Input: dimensioned drawing with shaded views. Units: mm. Origin: part minimum x, y, z. A direction names the side the tool comes from. Give positions to 0.01 mm unless a question says otherwise; leave off trailing zeros. Write each loop counter-clockwise with the first axis right and the second up, starting at its lowest first coordinate (ties: lowest second). Pieces come first, ordered by that corner, then holes. Notation, with made-up numbers: M -22,78.5 L 14,78.5 A21 ccw 14,86.5 Z; hole C 18,-15.5 d9. An arc over 180 degrees is marked long. Answer as a JSON object with one key per item and string values.
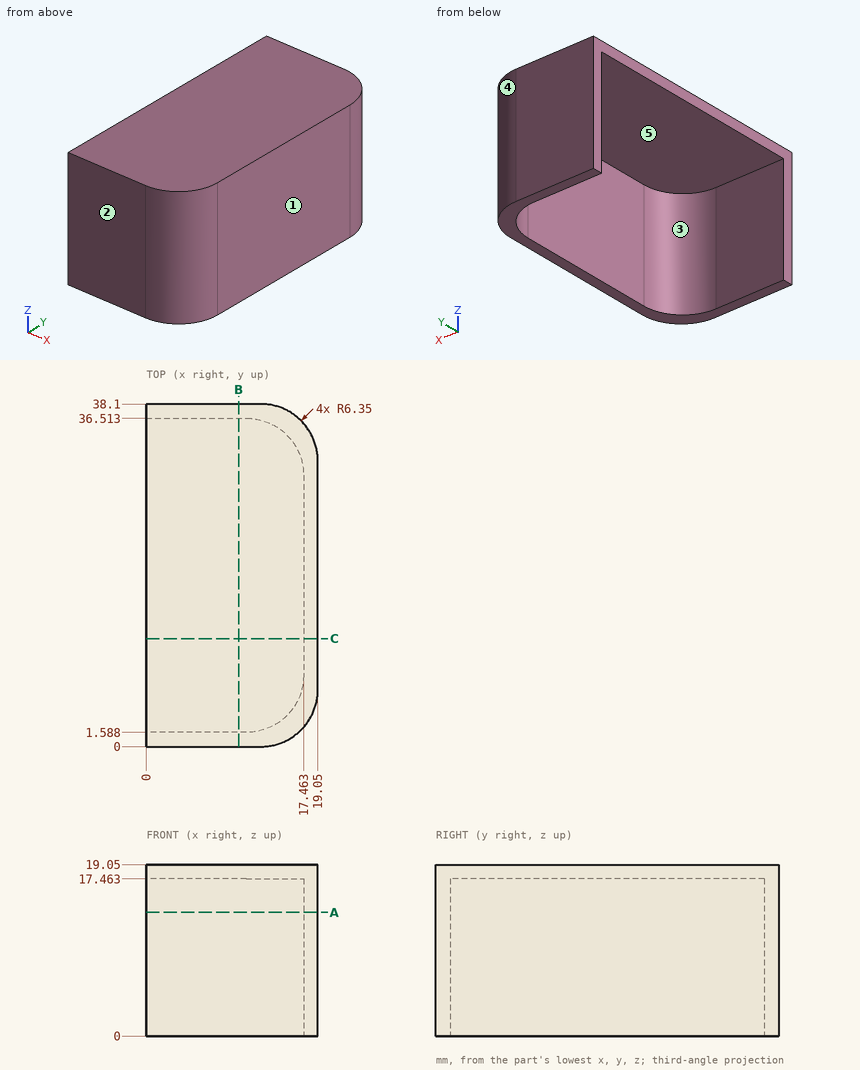
1) Set-up query: the marked faces 4 and 5. Return all of +Z, -Z, +X, -X, +Y, -Y with unobstructed straight access to the full face (end or side cutting, diameter ignored); none if empty.
Geometry check:
{"face 4": "+Z, -Z, +X, +Y", "face 5": "-Z, -X"}
2) Pull-direction query (Y, two-part tool) for the marked faces 1, 2 and 3; classes: pulls with the +Y half, pulls with the -Y half, needs draft (parallel to the pull), parting line crosses it, or undercut.
Geometry check:
{"face 1": "needs draft", "face 2": "pulls with the -Y half", "face 3": "undercut"}
3) Cut plane A-A on z = 13.75. Return loops of the section in (x, y).
Geometry check:
{"outline": "M 0,0 L 12.7,0 A6.35 ccw 19.05,6.35 L 19.05,31.75 A6.35 ccw 12.7,38.1 L 0,38.1 L 0,36.51 L 11.11,36.51 A6.35 cw 17.46,30.16 L 17.46,7.94 A6.35 cw 11.11,1.59 L 0,1.59 Z"}
4) Line query: line 1 (Y direction, x = 9.5, z = 9.5); line 2 (Z direction, x = 16.75, y = 27). Output: solid intervals per line, ascending. Write a range as from..to.
Geometry check:
{"line 1": "y = 0..1.59, 36.51..38.1", "line 2": "z = 17.46..19.05"}
5) Contact query for flat-ended pins moving along their axis: P1, Ø3, axis at y = 19, z = 15.5, coming from the -X side; P2, Ø4, axis at y = 33.5, z = 11.5, coming from the +X side; P3, Ø5, axis at x = 15.5, z = 16, coming from the -Y side; P4, Ø2, axis at x = 15.5, y = 5, coming from the -Z side. Output: stop coordinate, or through.
Geometry check:
{"P1": "stops at x = 17.46", "P2": "stops at x = 19.05", "P3": "stops at y = 0.01", "P4": "stops at z = 17.46"}
6) Cut plane C-C on y = 12. Return loops of the section in (x, z).
Geometry check:
{"outline": "M 0,17.46 L 17.46,17.46 L 17.46,0 L 19.05,0 L 19.05,19.05 L 0,19.05 Z"}
7) Cut plane B-B on x = 10.25. Return loops of the section in (y, z), and give its area (3 significant figures).
Geometry check:
{"outline": "M 0,0 L 1.59,0 L 1.59,17.46 L 36.51,17.46 L 36.51,0 L 38.1,0 L 38.1,19.05 L 0,19.05 Z", "area": "116 mm2"}
